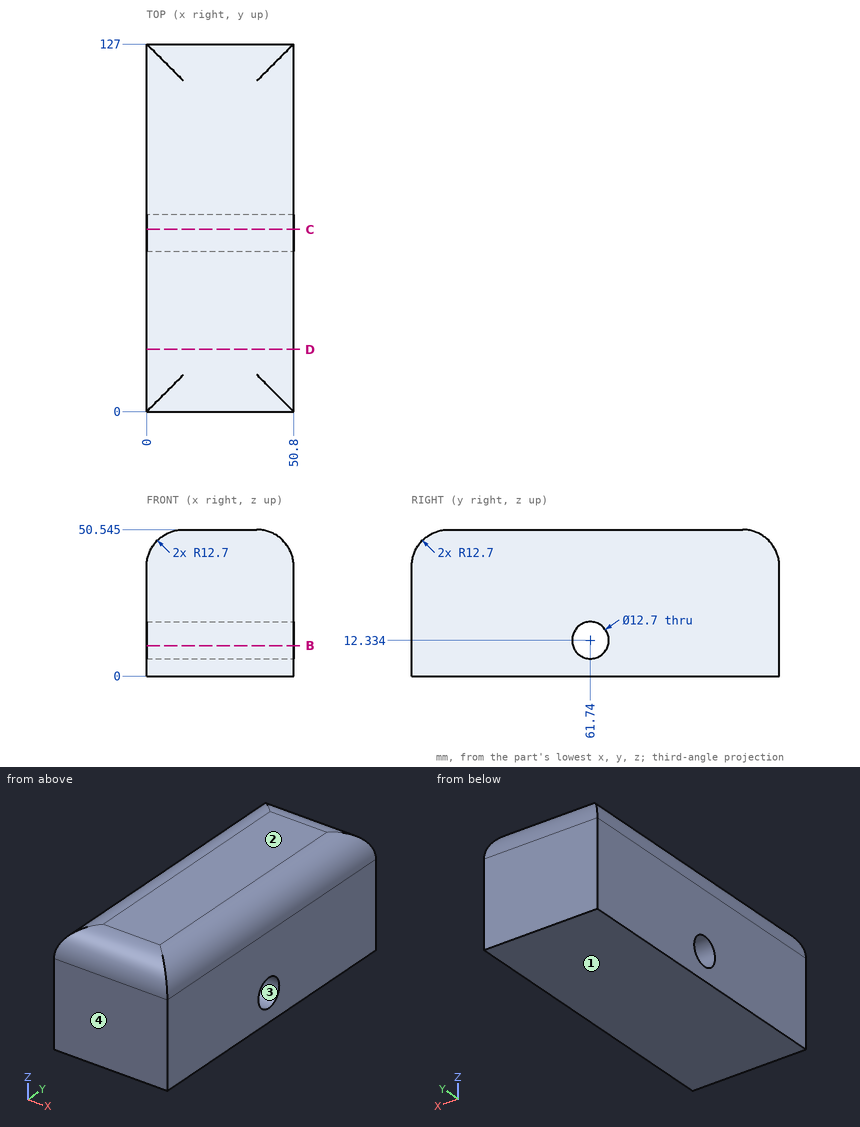
Source: three-view drawing plus pictorial views. Frame: mm from the lowest corner of the part. Coordinates: 2 decimals unless noted, no trailing zeros. Order: outer loops, then holes, each group sorted by start corner. A loop starts at its lowest first (then second) coordinate and runs counter-clockwise, first axis right, second up. Notation, with made-up numbers: M 32.5,66.5 L 43.5,66.5 A17 ccw 43.5,94.5 Z; hole C -18,83 d8. An arc over 180 degrees is marked long. One line per question, with ' | ' between items. Start each with the question number.
Item 1: Pin query (flat end, axial travel): pin 1 Ø11.5 at (y, z) = (61.74, 12.33) entering from -X; pin 2 Ø1.5 at (x, y) = (29, 101) entering from -Z. Return the tip coordinate at first contact, or that it passes through.
Item 2: Ray query, probe 1 along Z at (x, y) = (18, 58.5) (1 decimal); probe 2 along Y at (x, z) = (39, 9) (1 decimal); probe 3 along X at (y, z) = (99, 38). Return the intervals inside material, ascending. Write a range as [from, to].
Item 3: Cut plane D-D, the plane y = 21.5. Return the cut outline in (x, z) (1 decimal).
Item 4: Cut plane C-C, the plane y = 63. Return the cut outline in (x, z) (1 decimal).
Item 5: Cut plane B-B, the plane z = 10.5. Return the cut outline in (x, y).
Item 6: Draft query along Z for the marked faces 1, 2, 3 and 4. Return one class per face: released by +Z, released by -Z, zero draft, split by the parting line, or undercut.
A:
1) pin 1: passes through | pin 2: stops at z = 0
2) probe 1: z = [0, 6.9], [17.8, 50.5] | probe 2: y = [0, 56.3], [67.1, 127] | probe 3: x = [0, 50.8]
3) outline: M 0,0 L 50.8,0 L 50.8,37.8 A12.7 ccw 38.1,50.5 L 12.7,50.5 A12.7 ccw 0,37.8 Z
4) outline: M 0,0 L 50.8,0 L 50.8,6.1 L 0,6.1 Z; M 0,18.6 L 50.8,18.6 L 50.8,37.8 A12.7 ccw 38.1,50.5 L 12.7,50.5 A12.7 ccw 0,37.8 Z
5) outline: M 0,0 L 50.8,0 L 50.8,55.66 L 0,55.66 Z; M 0,67.82 L 50.8,67.82 L 50.8,127 L 0,127 Z
6) face 1: released by -Z | face 2: released by +Z | face 3: undercut | face 4: zero draft
